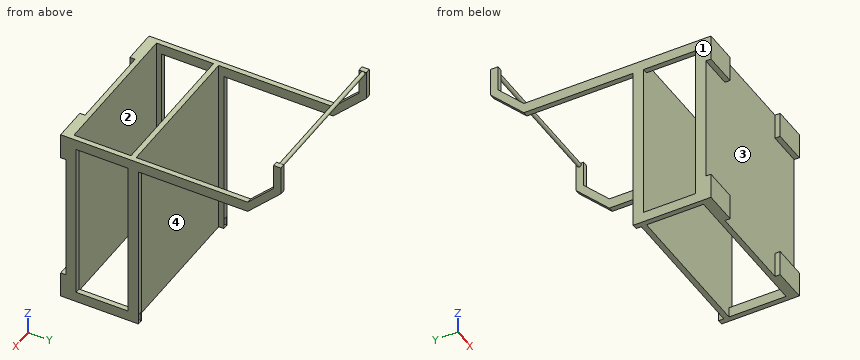
from build123d import *

# Parameters (mm, degrees)
EXTRUDE_THIN1_START             = 100
EXTRUDE_THIN1_OUTLINE_W         = 20
EXTRUDE_THIN1_OUTLINE_H         = 40
EXTRUDE_THIN1_OUTLINE_W_2       = 18
EXTRUDE_THIN1_OUTLINE_H_2       = 38
EXTRUDE_THIN1_DEPTH             = 701.72
SKETCH5_W                       = 20
SKETCH5_H                       = 40
SKETCH5_W_2                     = 18
SKETCH5_H_2                     = 38
EXTRUDE_THIN2_DEPTH             = 620
SKETCH6_W                       = 20
SKETCH6_H                       = 421.72
CUT_EXTRUDE1_DEPTH              = 1081.904694411
BOSS_EXTRUDE1_REACH             = 1107.783
SKETCH8_W                       = 700
SKETCH8_H                       = 20
BOSS_EXTRUDE1_DIRECTION_2_REACH = 1107.783
BOSS_EXTRUDE2_REACH             = 1214.087
SKETCH9_W                       = 700
SKETCH9_H                       = 20
BOSS_EXTRUDE3_DEPTH             = 20
BOSS_EXTRUDE4_DEPTH             = 20
BOSS_EXTRUDE5_REACH             = 1311.545
SKETCH12_R                      = 7.5
SKETCH16_W                      = 130
SKETCH16_H                      = 100
BOSS_EXTRUDE6_DEPTH             = 20


# Read off the part's stored shape, not the designer's step: Extrude-Thin1
with BuildPart() as part:
    # Extrude-Thin1 outline → Extrude-Thin1 (new body)
    # profile 1 of 4: a face of its own
    with BuildSketch(Plane(origin=(0, 0, 0), x_dir=(1, 0, 0), z_dir=(0, 1, 0)).offset(EXTRUDE_THIN1_START)):
        with Locations((-290, 680)):
            Rectangle(EXTRUDE_THIN1_OUTLINE_W, EXTRUDE_THIN1_OUTLINE_H)
        with Locations((-290, 680)):
            Rectangle(EXTRUDE_THIN1_OUTLINE_W_2, EXTRUDE_THIN1_OUTLINE_H_2, mode=Mode.SUBTRACT)
    # profile 2 of 4: a face of its own
    with BuildSketch(Plane(origin=(0, 0, 0), x_dir=(1, 0, 0), z_dir=(0, 1, 0)).offset(EXTRUDE_THIN1_START)):
        with Locations((290, 680)):
            Rectangle(EXTRUDE_THIN1_OUTLINE_W, EXTRUDE_THIN1_OUTLINE_H)
        with Locations((290, 680)):
            Rectangle(EXTRUDE_THIN1_OUTLINE_W_2, EXTRUDE_THIN1_OUTLINE_H_2, mode=Mode.SUBTRACT)
    # profile 3 of 4: a face of its own
    with BuildSketch(Plane(origin=(0, 0, 0), x_dir=(1, 0, 0), z_dir=(0, 1, 0)).offset(EXTRUDE_THIN1_START)):
        with Locations((290, 20)):
            Rectangle(EXTRUDE_THIN1_OUTLINE_W, EXTRUDE_THIN1_OUTLINE_H)
        with Locations((290, 20)):
            Rectangle(EXTRUDE_THIN1_OUTLINE_W_2, EXTRUDE_THIN1_OUTLINE_H_2, mode=Mode.SUBTRACT)
    # profile 4 of 4: a face of its own
    with BuildSketch(Plane(origin=(0, 0, 0), x_dir=(1, 0, 0), z_dir=(0, 1, 0)).offset(EXTRUDE_THIN1_START)):
        with Locations((-290, 20)):
            Rectangle(EXTRUDE_THIN1_OUTLINE_W, EXTRUDE_THIN1_OUTLINE_H)
        with Locations((-290, 20)):
            Rectangle(EXTRUDE_THIN1_OUTLINE_W_2, EXTRUDE_THIN1_OUTLINE_H_2, mode=Mode.SUBTRACT)
    extrude(amount=EXTRUDE_THIN1_DEPTH)

    # Sketch5 → Extrude-Thin2 (add)
    # profile 1 of 4: a face of its own
    with BuildSketch(Plane.XY.offset(-660)):
        with Locations((-290, 360)):
            Rectangle(SKETCH5_W, SKETCH5_H)
        with Locations((-290, 360)):
            Rectangle(SKETCH5_W_2, SKETCH5_H_2, mode=Mode.SUBTRACT)
    # profile 2 of 4: a face of its own
    with BuildSketch(Plane.XY.offset(-660)):
        with Locations((290, 360)):
            Rectangle(SKETCH5_W, SKETCH5_H)
        with Locations((290, 360)):
            Rectangle(SKETCH5_W_2, SKETCH5_H_2, mode=Mode.SUBTRACT)
    # profile 3 of 4: a face of its own
    with BuildSketch(Plane.XY.offset(-660)):
        with Locations((-290, 120)):
            Rectangle(SKETCH5_W, SKETCH5_H)
        with Locations((-290, 120)):
            Rectangle(SKETCH5_W_2, SKETCH5_H_2, mode=Mode.SUBTRACT)
    # profile 4 of 4: a face of its own
    with BuildSketch(Plane.XY.offset(-660)):
        with Locations((290, 120)):
            Rectangle(SKETCH5_W, SKETCH5_H)
        with Locations((290, 120)):
            Rectangle(SKETCH5_W_2, SKETCH5_H_2, mode=Mode.SUBTRACT)
    extrude(amount=EXTRUDE_THIN2_DEPTH)

    # Sketch6 → Cut-Extrude1 (cut, through all)
    with BuildSketch(Plane.XY.offset(-660)):
        with Locations((290, 590.86)):
            Rectangle(SKETCH6_W, SKETCH6_H)
        with Locations((-290, 590.86)):
            Rectangle(SKETCH6_W, SKETCH6_H)
    extrude(amount=-CUT_EXTRUDE1_DEPTH, mode=Mode.SUBTRACT)

    # Sketch8 → Boss-Extrude1 (add, up to next)
    with BuildSketch(Plane(origin=(0, 0, 0), x_dir=(0, 0, -1), z_dir=(1, 0, 0)), mode=Mode.PRIVATE) as boss_extrude1_sk1:
        with Locations((350, 350)):
            Rectangle(SKETCH8_W, SKETCH8_H)
    boss_extrude1_tool1 = extrude(boss_extrude1_sk1.sketch, amount=BOSS_EXTRUDE1_REACH, mode=Mode.PRIVATE) - part.part
    add(boss_extrude1_tool1.solids().sort_by_distance((0, 350, -350))[0])

    # Sketch8 → Boss-Extrude1 direction 2 (add, up to next)
    with BuildSketch(Plane(origin=(0, 0, 0), x_dir=(0, 0, -1), z_dir=(1, 0, 0)), mode=Mode.PRIVATE) as boss_extrude1_direction_2_sk1:
        with Locations((350, 350)):
            Rectangle(SKETCH8_W, SKETCH8_H)
    boss_extrude1_direction_2_tool1 = extrude(boss_extrude1_direction_2_sk1.sketch, amount=-BOSS_EXTRUDE1_DIRECTION_2_REACH, mode=Mode.PRIVATE) - part.part
    add(boss_extrude1_direction_2_tool1.solids().sort_by_distance((0, 350, -350))[0])

    # Sketch9 → Boss-Extrude2 (add, up to next)
    with BuildSketch(Plane.ZY.offset(-280), mode=Mode.PRIVATE) as boss_extrude2_sk1:
        with Locations((-350, 110)):
            Rectangle(SKETCH9_W, SKETCH9_H)
    boss_extrude2_tool1 = extrude(boss_extrude2_sk1.sketch, amount=BOSS_EXTRUDE2_REACH, mode=Mode.PRIVATE) - part.part
    add(boss_extrude2_tool1.solids().sort_by_distance((280, 110, -350))[0])

    # Sketch10 → Boss-Extrude3 (add)
    with BuildSketch(Plane(origin=(300, 0, 0), x_dir=(0, 0, -1), z_dir=(1, 0, 0))):
        Polygon((-200, 901.72), (-100, 901.72), (0, 801.72), (40, 801.72), (-88.284271247, 930.004271247), (-200, 930.004271247), align=None)
    extrude(amount=-BOSS_EXTRUDE3_DEPTH)

    # Sketch11 → Boss-Extrude4 (add)
    with BuildSketch(Plane.ZY.offset(300)):
        Polygon((-40, 801.72), (0, 801.72), (100, 901.72), (200, 901.72), (200, 930.004271247), (88.284271247, 930.004271247), align=None)
    extrude(amount=-BOSS_EXTRUDE4_DEPTH)

    # Sketch12 → Boss-Extrude5 (add, up to next)
    with BuildSketch(Plane(origin=(300, 0, 0), x_dir=(0, 0, -1), z_dir=(1, 0, 0)), mode=Mode.PRIVATE) as boss_extrude5_sk1:
        with Locations(Location((-192.5, 917.504271247, 0), (0, 0, 180))):
            Circle(SKETCH12_R)
    boss_extrude5_tool1 = extrude(boss_extrude5_sk1.sketch, amount=-BOSS_EXTRUDE5_REACH, mode=Mode.PRIVATE) - part.part
    add(boss_extrude5_tool1.solids().sort_by_distance((300, 917.504271, 192.5))[0])

    # Sketch16 → Boss-Extrude6 (add)
    with BuildSketch(Plane.XZ.offset(-100)):
        with Locations((-235, -50)):
            Rectangle(SKETCH16_W, SKETCH16_H)
        with Locations((235, -50)):
            Rectangle(SKETCH16_W, SKETCH16_H)
        with Locations((235, -650)):
            Rectangle(SKETCH16_W, SKETCH16_H)
        with Locations((-235, -650)):
            Rectangle(SKETCH16_W, SKETCH16_H)
    extrude(amount=BOSS_EXTRUDE6_DEPTH)


solid = part.part
Input: part model. Units: mm. Frame: model coordinates. Face numbers are marked on the shaded views. A direction names the side the tool comes from. Round coordinates to 2 decimals unless told otherwise and drop trailing zeros. Write each loop counter-clockwise with the first axis right and the second up, starting at its lowest first coordinate (ties: lowest second). Pieces come first, ordered by that corner, then holes.
1) Cut plane D-D (y = 734). Return the cut outline in (x, z), then the cut area to 3 significant figures.
2) Ray query, L1, parallel to Y at x = 131.5, z = -0.5; L2, parallel to Y at x = -259.5, z = -88. Return the intervals inside material, ascending.
3) Cut plane C-C (z = 128). Return the cut outline in (x, y), then the cut area to 3 significant figures.
4) Draft query along Z for the marked faces 3 and 4. Return one class per face: pulls with the +Z half, pulls with the -Z half, needs draft (parallel to the pull), parting line crosses it, or undercut.
5) Contact query for flat-ended pins moving along their axis: P1, Ø20, axis at x = 287.5, z = -19.5, coming from the +Y side; P2, Ø3, axis at x = -36, z = -157.5, coming from the +Y side; P3, Ø12, axis at x = -49, z = -64.5, coming from the -Y side. Output: stop coordinate, or through.
6) Cut plane A-A (y = 263). Count the separate pieces of the cut face and the enclosed holes in it, then the cut area to 3 significant figures.
7) Reachability of the marked faces 1 and 2 from +Z, -Z, +X, -X, +Y, -Y: full face, straight path, thin tool, end or side. Return the list, or none.
Geometry says:
1. outline: (-300, -40) - (-280, -40) - (-280, 0) - (-300, 0) - close; (280, -40) - (300, -40) - (300, 0) - (280, 0) - close; hole (-299, -39) - (-281, -39) - (-281, -1) - (-299, -1) - close; hole (281, -39) - (299, -39) - (299, -1) - (281, -1) - close
1. area: 232 mm2
2. L1: y = 100 to 120, 340 to 360
2. L2: y = 80 to 120, 340 to 360
3. outline: (-300, 901.72) - (-280, 901.72) - (-280, 930) - (-300, 930) - close; (280, 901.72) - (300, 901.72) - (300, 930) - (280, 930) - close
3. area: 1,130 mm2
4. face 3: undercut
4. face 4: needs draft
5. P1: stops at y = 832.22
5. P2: stops at y = 360
5. P3: stops at y = 100
6. separate pieces: 4
6. enclosed holes: 4
6. area: 464 mm2
7. face 1: +Z, -Z, -X, +Y, -Y
7. face 2: +Z, -Z
